Check sheet for the modelled part. Datum: model origin and axes. Units: mm. A direction names the side the tool comes from. Round coordinates to 2 decimals unless told otherwise and drop trailing zeros. Order: outer loops, then holes, each group sorted by start corner. A loop starts at its lowest first (then second) coordinate and runs counter-clockwise, first axis right, second up.
Q1. Cross-section at C-C on x = 10.25. Record the cut outline in (y, z), then the cut area to 3 significant figures.
Q2. Mould release check, pull along Y, two halves, no side actions. Record for faces 1 (the cylindrical face through (-1.183, 19.884, 5.247)), 2 (the cylindrical face through (0.6, 41.93, 5.06)), 3 (the flat face through (-2.4, 22, 5)): +Y half, -Y half, draft (parallel to the pull), parting line (faces both ways), or undercut.
Q3. Cross-section at B-B on z = 5. Record the cut outline in (x, y).
Q4. Cross-section at D-D on z = 8. Record the cut outline in (x, y).
Q5. Scan lines: probe 1 along Y at (x, z) = (-0.55, 5); probe 2 along X at (y, z) = (19, 0.5); probe 3 along Y at (x, z) = (4.5, 7.25). Record each from-to range of solid material in increasing order.
Q6. Depth check by flat-ended pin: P1, Ø1.8, axis at x = -4, z = 6.5, coming from the -Y side; P2, Ø3.5, axis at y = 8, z = 5, coming from the -X side; P3, Ø6, axis at y = 18, z = 5, coming from the +X side; P4, Ø3, axis at y = 39.5, z = 1.5, coming from the +X side. Enter the tip coordinate at first touch or a pass-through.
Q7. Cross-section at A-A on y = 8. Record the cut outline in (x, z).
Q8. Set-up check for faces 4 (the flat face through (0, 21, 5)), 5 (the flat face through (-4, 44, 5)), 6 (the flat face through (-0.2, 21.8, 0.2)), 7 (the flat face through (5.68, 42.62, 9.72)): record each of +Z, -Z, +X, -X, +Y, -Y from which the full face is reachable in a straight line by a thin tool's end or side.
Autodesk Inventor part; units mm, degrees
ref_plane "YZ Plane" through (0, 0, 0) normal (1, 0, 0) x (0, 1, 0)
ref_plane "XZ Plane" through (0, 0, 0) normal (0, 1, 0) x (-1, 0, 0)
ref_plane "XY Plane" through (0, 0, 0) normal (0, 0, 1) x (1, 0, 0)
sketch "Sketch1" plane through (0, 0, 0) normal (0, 0, 1) x (1, 0, 0)
  line L0 (-2.4, 0) -> (-2.4, 44)
  line L1 (-2.4, 44) -> (-4.7, 44)
  line L2 (-4.7, 44) -> (-6.4, 42)
  line L3 (-6.4, 42) -> (-6.8, 42)
  line L4 (-6.8, 42) -> (-6.8, 46.5)
  line L5 (-6.8, 46.5) -> (12, 46.5)
  line L6 (12, 46.5) -> (12, 42.5)
  line L7 (12, 42.5) -> (0, 42.5)
  line L8 (0, 42.5) -> (0, 0)
  line L9 (0, 0) -> (-2.4, 0)
  dimension "d0" = 44
  dimension "d3" = 2.4
  dimension "d5" = 2.5
  dimension "d6" = 4
  dimension "d7" = 12
  dimension "d19" = 18.8
  dimension "d20" = 0.4
  dimension "d21" = 2
  dimension "d22" = 2.3
extrude "Extrusion1" add sketch "Sketch1" along normal blind 10
sketch "Sketch2" plane through (0, 0, 0) normal (1, 0, 0) x (0, 0, -1)
  circle A0 centre (-5, 8) radius 1.9
  line L0 (0, 0) -> (-10, 0)
  line L1 (-10, 0) -> (-10, 42.5)
  line L2 (0, 42.5) -> (-10, 42.5)
  circle A1 centre (-5, 18) radius 1.9
  dimension "d10" = 3.8
  dimension "d11" = 8
  dimension "d12" = 5
  dimension "d23" = 34.5
  dimension "d26" = 10
extrude "Extrusion3" cut sketch "Sketch2" against normal through all
chamfer "Chamfer1" distance 0.4 angle 45 19 edges at (0, 21.25, 10) (0, 0, 5) (0, 21.25, 0) (6, 42.5, 0) (6, 42.5, 10) (12, 42.5, 5) (12, 46.5, 5) (12, 44.5, 10) (12, 44.5, 0) (-6.8, 46.5, 5) (2.6, 46.5, 10) (2.6, 46.5, 0) (-6.8, 44.25, 0) (-6.8, 44.25, 10) (-2.4, 22, 0) (-2.4, 0, 5) (-2.4, 22, 10) (-3.55, 44, 10) (-3.55, 44, 0)
fillet "Fillet1" radius 2 1 edges at (0, 42.5, 5)
properties part number "Battery Latch"
Results found:
1. outline: (42.5, 0.4) - (42.9, 0) - (46.1, 0) - (46.5, 0.4) - (46.5, 9.6) - (46.1, 10) - (42.9, 10) - (42.5, 9.6) - close
1. area: 39.7 mm2
2. face 1: undercut
2. face 2: -Y half
2. face 3: draft
3. outline: (-6.8, 42) - (-6.4, 42) - (-4.7, 44) - (-2.4, 44) - (-2.4, 19.9) - (0, 19.9) - (0, 40.5) arc R2 cw to (2, 42.5) - (11.6, 42.5) - (12, 42.9) - (12, 46.1) - (11.6, 46.5) - (-6.4, 46.5) - (-6.8, 46.1) - close; (-2.4, 0.4) - (-2, 0) - (-0.4, 0) - (0, 0.4) - (0, 6.1) - (-2.4, 6.1) - close; (-2.4, 9.9) - (0, 9.9) - (0, 16.1) - (-2.4, 16.1) - close
4. outline: (-6.8, 42) - (-6.4, 42) - (-4.7, 44) - (-2.4, 44) - (-2.4, 0.4) - (-2, 0) - (-0.4, 0) - (0, 0.4) - (0, 40.5) arc R2 cw to (2, 42.5) - (11.6, 42.5) - (12, 42.9) - (12, 46.1) - (11.6, 46.5) - (-6.4, 46.5) - (-6.8, 46.1) - close
5. probe 1: y = 0 to 6.1, 9.9 to 16.1, 19.9 to 46.5
5. probe 2: x = -2.4 to 0
5. probe 3: y = 42.5 to 46.5
6. P1: stops at y = 43.76
6. P2: passes through
6. P3: stops at x = 0
6. P4: stops at x = 0.06
7. outline: (-2.4, 0.4) - (-2, 0) - (-0.4, 0) - (0, 0.4) - (0, 3.1) - (-2.4, 3.1) - close; (-2.4, 6.9) - (0, 6.9) - (0, 9.6) - (-0.4, 10) - (-2, 10) - (-2.4, 9.6) - close
8. face 4: +Z, -Z, +X, -Y
8. face 5: +Z, -Z, -Y
8. face 6: -Z, +X, -Y
8. face 7: +Z, +X, -Y
